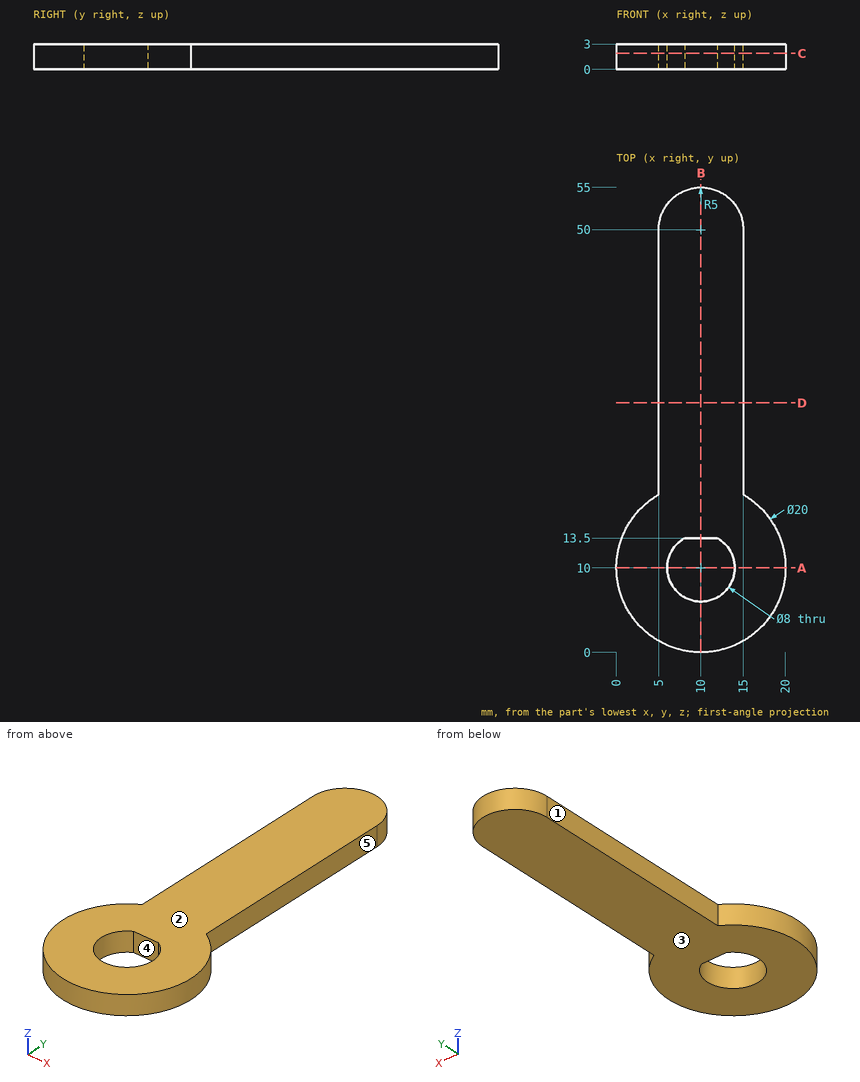
Job drawing, mm, ordinate dimensions from the low corner. One solid piece. A direction names the side the tool comes from. Coordinates: 2 decimals unless noted, no trailing zeros. Write each loop counter-clockwise with the first axis right and the second up, starting at its lowest first coordinate (ties: lowest second). Pieces come first, ordered by that corner, then holes.
Item 1: Probe line 1 (X direction, y = 46, z = 1); line 2 (Y direction, x = 9, z = 0.5); line 3 (Y direction, x = 12, z = 0.25). List the from-to ranges inside material, lowest first.
Item 2: Pin check, flat tips, straight feed: pin 1 (1.5 mm diameter, centred on y = 46, z = 1, fed in from +X); pin 2 (1.5 mm diameter, centred on x = 13.5, z = 1.5, fed in from -Y); pin 3 (0.9 mm diameter, centred on y = 34.5, z = 1.5, fed in from -X). Stop position of each tip, or through.
Item 3: Slice it at A-A (y = 10). Write the cut outline in (x, z).
Item 4: Which spindle directions (+Z, -Z, +X, -X, +Y, -Y) get a long thin tool onto all of the face, cutting with end or side? Do the marked faces 1 and 2. Say none if no direction does.
Item 5: Slice it at B-B (x = 10). Write the cut outline in (y, z), and give its area (4 significant figures).
Item 6: Mould opens along X. For the marked faces 3, 4 and 5 say: released by +X, released by -X, zero draft, split by the parting line, or undercut.
Item 7: Slice it at C-C (z = 1.9). Write the cut outline in (x, y), and give its area (3 significant figures).
Item 8: Slice it at D-D (y = 29.5). Write the cut outline in (x, z).
Results found:
1. line 1: x = 5 to 15
1. line 2: y = 0.05 to 6.13, 13.5 to 54.9
1. line 3: y = 0.2 to 6.54, 13.46 to 54.58
2. pin 1: stops at x = 15
2. pin 2: stops at y = 0.39
2. pin 3: stops at x = 5
3. outline: (0, 0) - (6, 0) - (6, 3) - (0, 3) - close; (14, 0) - (20, 0) - (20, 3) - (14, 3) - close
4. face 1: +Z, -Z, -X, +Y
4. face 2: +Z, +X, -X, +Y, -Y
5. outline: (0, 0) - (6, 0) - (6, 3) - (0, 3) - close; (13.5, 0) - (55, 0) - (55, 3) - (13.5, 3) - close
5. area: 142.5 mm2
6. face 3: zero draft
6. face 4: undercut
6. face 5: released by +X
7. outline: (5, 18.66) arc R10 ccw (long way) to (15, 18.66) - (15, 50) arc R5 ccw to (5, 50) - close; hole (8.06, 13.5) arc R4 ccw (long way) to (11.94, 13.5) - close
7. area: 609 mm2
8. outline: (5, 0) - (15, 0) - (15, 3) - (5, 3) - close
